from build123d import *
from build123d.topology import SkipClean

# Parameters (mm, degrees)
SKETCH_1_R          = 11.75
EXTRUDE_1_DEPTH     = 3
CUT_EXTRUDE_1_DEPTH = 13
SKETCH_3_R          = 10.2
SKETCH_3_R_2        = 7
CUT_EXTRUDE_2_DEPTH = 1.6
EXTRUDE_START       = 1.5
EXTRUDE_2_DEPTH     = 1.5
FILLET_1_R          = 1.5
EXTRUDE_START_2     = 2
SKETCH_7_R          = 4.4
EXTRUDE_4_DEPTH     = 2
EXTRUDE_START_3     = 19
SKETCH_9_R          = 4.4
EXTRUDE_5_DEPTH     = 19
SKETCH_10_W         = 6
SKETCH_10_H         = 6
EXTRUDE_6_DEPTH     = 5
CUT_EXTRUDE_START   = -10
CUT_EXTRUDE_4_DEPTH = 10


with BuildPart() as part:
    # 草图1 → 凸台-拉伸1 (new body)
    with BuildSketch(Plane.XY):
        Circle(SKETCH_1_R)
    extrude(amount=EXTRUDE_1_DEPTH)

    # 草图2 → 切除-拉伸1 (cut)
    with BuildSketch(Plane(origin=(0, 0, 0), x_dir=(-1, 0, 0), z_dir=(0, 0, -1))):
        with BuildLine():
            Line((1.429160593, -0.6), (-1.429160593, -0.6))
            ThreePointArc((-1.429160593, -0.6), (0, 1.55), (1.429160593, -0.6))
        make_face()
    extrude(amount=-CUT_EXTRUDE_1_DEPTH, mode=Mode.SUBTRACT)

    # 草图3 → 切除-拉伸2 (cut)
    with BuildSketch(Plane.XY.offset(3)):
        Circle(SKETCH_3_R)
        Circle(SKETCH_3_R_2, mode=Mode.SUBTRACT)
    extrude(amount=-CUT_EXTRUDE_2_DEPTH, mode=Mode.SUBTRACT)

    # 草图4 → 凸台-拉伸2 (add)
    with BuildSketch(Plane.XY.offset(1.4).offset(EXTRUDE_START)):
        with BuildLine():
            Line((1.811733316, -6.761480784), (2.63995426, -9.852443428))
            ThreePointArc((2.63995426, -9.852443428), (0, -10.2), (-2.63995426, -9.852443428))
            Line((-2.63995426, -9.852443428), (-1.811733316, -6.761480784))
            ThreePointArc((-1.811733316, -6.761480784), (0, -7), (1.811733316, -6.761480784))
        make_face()
    extrude(amount=-EXTRUDE_2_DEPTH)

    # 圆角1
    fillet_1_edges = [part.edges().sort_by_distance(p)[0] for p in [
        (1.811733316, -6.761480784, 2.15),
        (-1.811733316, -6.761480784, 2.15),
        (-2.63995426, -9.852443428, 2.15),
        (2.63995426, -9.852443428, 2.15),
    ]]
    fillet(fillet_1_edges, radius=FILLET_1_R)

    # 草图7 → 凸台-拉伸4 (add)
    with SkipClean():  # the faces are left unmerged after this step: merging them gives an invalid solid
        with BuildSketch(Plane(origin=(0, 0, 0), x_dir=(-1, 0, 0), z_dir=(0, 0, -1)).offset(EXTRUDE_START_2)):
            with Locations(Location((0, 0, 0), (0, 0, 180))):
                Circle(SKETCH_7_R)
            with BuildLine():
                Line((-1.429160593, -0.6), (1.429160593, -0.6))
                ThreePointArc((1.429160593, -0.6), (0, 1.55), (-1.429160593, -0.6))
            make_face(mode=Mode.SUBTRACT)
        extrude(amount=-EXTRUDE_4_DEPTH)

    # 草图9 → 凸台-拉伸5 (add)
    with SkipClean():  # the faces are left unmerged after this step: merging them gives an invalid solid
        with BuildSketch(Plane(origin=(0, 0, -2), x_dir=(-1, 0, 0), z_dir=(0, 0, -1)).offset(EXTRUDE_START_3)):
            with Locations(Location((0, 0, 0), (0, 0, 180))):
                Circle(SKETCH_9_R)
        extrude(amount=-EXTRUDE_5_DEPTH)

    # 草图10 → 凸台-拉伸6 (add)
    with SkipClean():  # the faces are left unmerged after this step: merging them gives an invalid solid
        with BuildSketch(Plane(origin=(0, 0, -21), x_dir=(-1, 0, 0), z_dir=(0, 0, -1))):
            Rectangle(SKETCH_10_W, SKETCH_10_H)
        extrude(amount=EXTRUDE_6_DEPTH)

    # 草图11 → 切除-拉伸4 (cut)
    with BuildSketch(Plane.XY.offset(3).offset(CUT_EXTRUDE_START)):
        with BuildLine():
            Line((1.49415528, -0.7), (-1.49415528, -0.7))
            ThreePointArc((-1.49415528, -0.7), (0, 1.65), (1.49415528, -0.7))
        make_face()
        with BuildLine():
            Line((1.429160593, -0.6), (-1.429160593, -0.6))
            ThreePointArc((-1.429160593, -0.6), (0, 1.55), (1.429160593, -0.6))
        make_face(mode=Mode.SUBTRACT)
    extrude(amount=CUT_EXTRUDE_4_DEPTH, mode=Mode.SUBTRACT)


solid = part.part
Could you check a few things on this model? Use its own coordinates, in mm. A direction names the side the tool comes from. Round coordinates to 2 decimals unless told otherwise and drop trailing zeros. Order: outer loops, then holes, each group sorted by start corner. A loop starts at its lowest first (then second) coordinate and runs counter-clockwise, first axis right, second up. Notation, with made-up numbers: M 75,-12.5 L 93,-12.5 A23 cw 93,0.5 Z; hole C 13,53.5 d11. An arc over 180 degrees is marked long. One line per item, written item: value.
(1) I need wall thicknesses on line 1 along Y through (x, z) = (0, 1.85); line 2 along Z through (x, y) = (-9.25, 4.75); line 3 along Z through (x, y) = (-0.5, -8.75). Which ranges of each line are inside material? Lowest first, please. Write a range as from..to.
Ans:
line 1: y = -11.75..-0.7, 1.65..7, 10.2..11.75
line 2: z = 0..3
line 3: z = 0..2.9
(2) Imagine slicing it at C-C (z = -12). Write out the boundary of the cut face in (x, y).
Ans:
outline: C 0,0 d8.8
(3) If we mould it in two halves opening along X, with no side actions, what happens to faces 1 (the cylindrical face through (-0.573, -4.363, -10.647)), 2 (the flat face through (3, 0, -23)), 3 (the flat face through (0, 3, -23)), 4 (the cylindrical face through (-2.25, -7.07, 2.14))? For each: released by +X, released by -X, zero draft, split by the parting line, or undercut.
Ans:
face 1: split by the parting line
face 2: released by +X
face 3: zero draft
face 4: undercut
(4) Imagine slicing it at D-D (y = -3.75). Write out the boundary of the cut face in (x, z).
Ans:
outline: M -11.14,0 L -2.3,0 L -2.3,-21 L 2.3,-21 L 2.3,0 L 11.14,0 L 11.14,3 L 9.49,3 L 9.49,1.4 L 5.91,1.4 L 5.91,3 L -5.91,3 L -5.91,1.4 L -9.49,1.4 L -9.49,3 L -11.14,3 Z
(5) Imagine slicing it at A-A (x = 0). Write out the boundary of the cut face in (y, z).
Ans:
outline: M -11.75,0 L -4.4,0 L -4.4,-21 L -3,-21 L -3,-26 L 3,-26 L 3,-21 L 4.4,-21 L 4.4,0 L 11.75,0 L 11.75,3 L 10.2,3 L 10.2,1.4 L 7,1.4 L 7,3 L 1.65,3 L 1.65,-7 L 1.55,-7 L 1.55,-2 L -0.6,-2 L -0.6,-7 L -0.7,-7 L -0.7,3 L -7,3 L -7,2.9 L -10.2,2.9 L -10.2,3 L -11.75,3 Z
(6) Imagine slicing it at B-B (y = 0). Write out the boundary of the cut face in (x, z).
Ans:
outline: M -11.75,0 L -4.4,0 L -4.4,-21 L -3,-21 L -3,-26 L 3,-26 L 3,-21 L 4.4,-21 L 4.4,0 L 11.75,0 L 11.75,3 L 10.2,3 L 10.2,1.4 L 7,1.4 L 7,3 L 1.65,3 L 1.65,-7 L 1.55,-7 L 1.55,-2 L -1.55,-2 L -1.55,-7 L -1.65,-7 L -1.65,3 L -7,3 L -7,1.4 L -10.2,1.4 L -10.2,3 L -11.75,3 Z
(7) Which directions (+Z, -Z, +X, -X, +Y, -Y) give clear straight access to the entire face, cutting with the end or side of a thin tool? Please do faces 5 (the flat face through (0, -3, -23)), 6 (the flat face through (0, 0, -2)), 7 (the flat face through (5, 0, 0)).
Ans:
face 5: -Z, +X, -X, -Y
face 6: +Z
face 7: -Z
(8) I'm going to push flat-ended pins straight in: P1, Ø3, axis at x = -1, y = -8.5, coming from the +Z side; P2, Ø0.9, axis at x = 0.5, z = -3, coming from the +Y side; P3, Ø3, axis at y = 5.5, z = -6, coming from the +X side; P4, Ø5, axis at y = -8.5, z = -21.5, coming from the +X side. Where does each tip first touch, or does it pass through?
Ans:
P1: stops at z = 2.9
P2: stops at y = 4.4
P3: stops at x = 1.83
P4: passes through
